Model file for the job. Use its own axes, mm. Coordinates: 2 decimals unless noted, no trailing zeros. Write each loop counter-clockwise with the first axis right and the second up, starting at its lowest first coordinate (ties: lowest second). Pieces come first, ordered by that corner, then holes. Notation, with made-up numbers: M 67,13.25 L 91,13.25 A8 cw 91,18.25 Z; hole C 40,-15 d3. An arc over 180 degrees is marked long. Put each result on its own line as item: value. Start each with the question number.
Q1. Drill centre lines: line 1 along X through (y, z) = (5, 33.5); line 2 along X through (y, z) = (16.75, 32); line 3 along Z through (x, y) = (38, 12). Where is each one in solid material? Low to high.
Q2. Pull direction X, two halves, no side cores. Call faces 1 (the flat face through (44, 0, 33)), 2 (the flat face through (90, 9, 34)), 3 (the cylindrical face through (35.022, 9.633, 35.858)), 4 (the cylindrical face through (58.185, 9.633, 32.983)): pulls with the +X half, pulls with the -X half, needs draft (parallel to the pull), parting line crosses it, or undercut.
Q3. Cut at A-A (x = 54.25). Write the cut outline in (y, z), then the cut area to 3 significant figures.
Q4. Cut at C-C (x = 36). Write the cut outline in (y, z).
Q5. Cut at B-B (z = 33.5). Write the cut outline in (x, y), then the cut area to 3 significant figures.
```python
from build123d import *

# Parameters (mm, degrees)
SKETCH_1_W            = 90
SKETCH_1_H            = 67
EXTRUDE_1_DEPTH       = 19
HOLE_WIZARD_1_4_201_D = 5.1054
HOLE_WIZARD_3_8_161_D = 7.9375


with BuildPart() as part:
    # Эскиз1 → Бобышка-Вытянуть1 (new body)
    with BuildSketch(Plane(origin=(0, 0, 0), x_dir=(1, 0, 0), z_dir=(0, 1, 0))):
        with Locations((45, -33.5)):
            Rectangle(SKETCH_1_W, SKETCH_1_H)
    extrude(amount=EXTRUDE_1_DEPTH)

    # Отверстие обработанное метчиком 1/4-201 (through all)
    with Locations(Plane(origin=(36, 0, 33.5), x_dir=(0, 0, -1), z_dir=(0, -1, 0))):
        with Locations((0, 0)):
            Hole(HOLE_WIZARD_1_4_201_D / 2)

    # Отверстие обработанное метчиком 3/8-161 (through all)
    with Locations(Plane(origin=(54.25, 0, 33.5), x_dir=(0, 0, -1), z_dir=(0, -1, 0))):
        with Locations((0, 0)):
            Hole(HOLE_WIZARD_3_8_161_D / 2)


solid = part.part
```
Computed values:
1. line 1: 0 to 33.45, 38.55 to 50.28, 58.22 to 90
1. line 2: 0 to 33.93, 38.07 to 50.58, 57.92 to 90
1. line 3: 0 to 31.91, 35.09 to 67
2. face 1: needs draft
2. face 2: pulls with the +X half
2. face 3: undercut
2. face 4: undercut
3. outline: M 0,0 L 19,0 L 19,29.53 L 0,29.53 Z; M 0,37.47 L 19,37.47 L 19,67 L 0,67 Z
3. area: 1,120 mm2
4. outline: M 0,0 L 19,0 L 19,30.95 L 0,30.95 Z; M 0,36.05 L 19,36.05 L 19,67 L 0,67 Z
5. outline: M 0,0 L 33.45,0 L 33.45,19 L 0,19 Z; M 38.55,0 L 50.28,0 L 50.28,19 L 38.55,19 Z; M 58.22,0 L 90,0 L 90,19 L 58.22,19 Z
5. area: 1,460 mm2
